The model under review builds one solid part; all positions refer to its coordinate system, in mm. A direction names the side the tool comes from. Give positions to 0.01 mm unless a question says otherwise; leave off trailing zeros. Order: outer loops, then holes, each group sorted by start corner. A loop starts at its lowest first (then second) coordinate and runs counter-clockwise, first axis right, second up.
```python
from build123d import *

# Parameters (mm, degrees)
BOSS_EXTRUDE1_DEPTH = 10


with BuildPart() as part:
    # Sketch1 → Boss-Extrude1 (new body)
    with BuildSketch(Plane(origin=(0, 0, 0), x_dir=(0, 0, -1), z_dir=(1, 0, 0))):
        Polygon((0, 616), (230, 616), (230, 546), (0, 546), (0, 0), (380, 0), (380, 792), (145, 792), (145, 942), (0, 942), align=None)
        with BuildLine():
            ThreePointArc((67.5, 804.5), (95, 777), (122.5, 804.5))
            Line((122.5, 804.5), (122.5, 889.5))
            ThreePointArc((122.5, 889.5), (95, 917), (67.5, 889.5))
            Line((67.5, 889.5), (67.5, 804.5))
        make_face(mode=Mode.SUBTRACT)
    extrude(amount=BOSS_EXTRUDE1_DEPTH)


solid = part.part
```
Item 1: For line 1 (Y direction, x = 2, z = -126); line 2 (Y direction, x = 8.25, z = -234.5); line 3 (Y direction, x = 4, z = -191), list the stretches that pass through material, from the lowest coordinate up.
Values found:
line 1: y = 0 to 546, 616 to 942
line 2: y = 0 to 792
line 3: y = 0 to 546, 616 to 792
Item 2: Clearance check with flat-ended pins moving along their axes: pin 1 Ø3 at (x, z) = (3.5, -300.5) entering from +Y; pin 2 Ø1.5 at (x, z) = (3.5, -301) entering from -Y. State where each tip first meets the part, or that it passes through.
Values found:
pin 1: stops at y = 792
pin 2: stops at y = 0
Item 3: For faces 3 (the flat face through (10, 373, -187)), 4 (the cylindrical face through (4.93, 916.993, -95.605)), list the 3-axis set-ups (+Z, -Z, +X, -X, +Y, -Y) from which the entire face can be reached by the end or side of a thin tool; tool diameter is ignored.
Values found:
face 3: +Z, -Z, +X, +Y, -Y
face 4: +X, -X
Item 4: Take a section at D-D (y = 602.5). Give the boundary of the cut face in (x, z), and give its area (3 significant figures).
Values found:
outline: (0, -380) - (10, -380) - (10, -230) - (0, -230) - close
area: 1,500 mm2
Item 5: Take a section at C-C (z = -213.5). Give the boundary of the cut face in (x, y).
Values found:
outline: (0, 0) - (10, 0) - (10, 546) - (0, 546) - close; (0, 616) - (10, 616) - (10, 792) - (0, 792) - close
Item 6: Take a section at A-A (z = -95). Give the boundary of the cut face in (x, y).
Values found:
outline: (0, 0) - (10, 0) - (10, 546) - (0, 546) - close; (0, 616) - (10, 616) - (10, 777) - (0, 777) - close; (0, 917) - (10, 917) - (10, 942) - (0, 942) - close
Item 7: Draft analysis for pull direction Z (two halves, no side actions). For faces 1 (the flat face through (0, 373, -187)), 2 (the cylindrical face through (4.93, 777.007, -94.395)), state which applies: released by +Z, released by -Z, zero draft, split by the parting line, or undercut.
Values found:
face 1: zero draft
face 2: undercut
Item 8: Take a section at B-B (x = 2.5). Give the boundary of the cut face in (y, z), and give its area (3 significant figures).
Values found:
outline: (0, -380) - (792, -380) - (792, -145) - (942, -145) - (942, 0) - (616, 0) - (616, -230) - (546, -230) - (546, 0) - (0, 0) - close; hole (804.5, -122.5) - (889.5, -122.5) arc R27.5 ccw to (889.5, -67.5) - (804.5, -67.5) arc R27.5 ccw to start
area: 300,000 mm2
